from build123d import *

# Parameters (mm, degrees)
SKETCH1_R           = 1.6
BOSS_EXTRUDE1_DEPTH = 5


with BuildPart() as part:
    # Sketch1 → Boss-Extrude1 (new body)
    with BuildSketch(Plane(origin=(0, 0, 0), x_dir=(1, 0, 0), z_dir=(0, 1, 0))):
        with BuildLine():
            Line((0, 3.5), (125.5, 3.5))
            ThreePointArc((125.5, 3.5), (129, 0), (125.5, -3.5))
            Line((125.5, -3.5), (0, -3.5))
            ThreePointArc((0, -3.5), (-3.5, 0), (0, 3.5))
        make_face()
        Circle(SKETCH1_R, mode=Mode.SUBTRACT)
        with Locations((125.5, 0)):
            Circle(SKETCH1_R, mode=Mode.SUBTRACT)
    extrude(amount=BOSS_EXTRUDE1_DEPTH)


solid = part.part
Geometry: final body of the model. Coordinates: model frame, mm. Coordinates: 2 decimals unless noted, no trailing zeros. Order: outer loops, then holes, each group sorted by start corner. A loop starts at its lowest first (then second) coordinate and runs counter-clockwise, first axis right, second up.
(1) First-contact query: pin 1 (2.5 mm diameter, centred on x = 125.5, z = 0, fed in from -Y); pin 2 (3.5 mm diameter, centred on x = 0, z = 0, fed in from -Y). Flat tips, straight axial feed; report the tip coordinate or a pass-through.
(2) Material intervals for probe 1 along X at (y, z) = (2.2, 0); probe 2 along Z at (x, y) = (0, 3.1); probe 3 along X at (y, z) = (1.9, 1.25), sorted ascending.
(3) Section query A-A (z = 0). Return the cut outline in (x, y), plus the area to 4 significant figures.
(4) Draft query along Z for faces 1 (the face through (127.026, 2.465, -0.481)), 2 (the face through (64, 0, 0)), 3 (the face through (62, 2, -3.5)), 4 (the face through (129, 2, 0)). Return one class per face: pulls with the +Z half, pulls with the -Z half, needs draft (parallel to the pull), parting line crosses it, or undercut.
(5) Section query B-B (y = 1.95). Return the cut outline in (x, z), plus the area to 3 significant figures.
Solution:
1. pin 1: passes through
1. pin 2: stops at y = 0
2. probe 1: x = -3.5 to -1.6, 1.6 to 123.9, 127.1 to 129
2. probe 2: z = -3.5 to -1.6, 1.6 to 3.5
2. probe 3: x = -3.27 to -1, 1 to 124.5, 126.5 to 128.77
3. outline: (-3.5, 0) - (-1.6, 0) - (-1.6, 5) - (-3.5, 5) - close; (1.6, 0) - (123.9, 0) - (123.9, 5) - (1.6, 5) - close; (127.1, 0) - (129, 0) - (129, 5) - (127.1, 5) - close
3. area: 630.5 mm2
4. face 1: undercut
4. face 2: needs draft
4. face 3: pulls with the -Z half
4. face 4: parting line crosses it
5. outline: (0, -3.5) - (125.5, -3.5) arc R3.5 ccw to (125.5, 3.5) - (0, 3.5) arc R3.5 ccw to start; hole circle Ø3.2 at (0, 0); hole circle Ø3.2 at (125.5, 0)
5. area: 901 mm2
